Build history of the part. All positions in model axes, mm. A direction names the side the tool comes from. Round coordinates to 2 decimals unless told otherwise and drop trailing zeros. Loops run counter-clockwise (first coordinate to the right, second up) from the corner with the lowest first, then second, coordinate; pieces in that order, holes last. Notation, with made-up numbers: M 68,51.5 L 76,51.5 A23 cw 76,84.5 Z; hole C 51,-15.75 d4. An arc over 180 degrees is marked long. Use one line per item in the form item = value. Start each with the question number.
```python
from build123d import *

# Parameters (mm, degrees)
SKETCH_1_W           = 18.1
SKETCH_1_H           = 18.7
EXTRUDE_1_DEPTH      = 20
SKETCH_2_W           = 13.1
SKETCH_2_H           = 11
EXTRUDE_2_DEPTH      = 2
EXTRUDE_3_DEPTH      = 9.7
EXTRUDE_3_DEPTH_BACK = 40
FILLET_1_R           = 2.5
FILLET_2_R           = 0.5
CUT_EXTRUDE_1_DEPTH  = 49.539674531
SKETCH_5_R           = 6.105797263
CUT_EXTRUDE_2_DEPTH  = 1
SKETCH_6_R           = 6.02468661
CUT_EXTRUDE_3_DEPTH  = 1


with BuildPart() as part:
    # ｽｹｯﾁ1 → ﾎﾞｽ - 押し出し1 (new body)
    with BuildSketch(Plane.XY):
        with Locations((9.05, 9.35)):
            Rectangle(SKETCH_1_W, SKETCH_1_H)
    extrude(amount=EXTRUDE_1_DEPTH)

    # ｽｹｯﾁ2 → ﾎﾞｽ - 押し出し2 (add)
    with BuildSketch(Plane(origin=(0, 18.7, 0), x_dir=(1, 0, 0), z_dir=(0, 1, 0))):
        with Locations((9.05, -5.5)):
            Rectangle(SKETCH_2_W, SKETCH_2_H)
    extrude(amount=EXTRUDE_2_DEPTH)

    # ｽｹｯﾁ3 → ﾎﾞｽ - 押し出し3 (add, two sides: drawn at the far end of the back side and taken through both)
    with BuildSketch(Plane(origin=(0, 0, 0), x_dir=(-1, 0, 0), z_dir=(0, 0, -1)).offset(-EXTRUDE_3_DEPTH_BACK)):
        with BuildLine():
            ThreePointArc((-2.566319039, 9.311012343), (-2.144244303, 16.230296479), (-9.064933475, 15.831923002))
            ThreePointArc((-9.064933475, 15.831923002), (-15.903655717, 16.221032622), (-15.521168651, 9.381936787))
            ThreePointArc((-15.521168651, 9.381936787), (-15.948030787, 2.480748206), (-9.045010779, 2.876891972))
            ThreePointArc((-9.045010779, 2.876891972), (-2.204371262, 2.467711109), (-2.566319039, 9.311012343))
        make_face()
    extrude(amount=EXTRUDE_3_DEPTH + EXTRUDE_3_DEPTH_BACK)

    # ﾌｨﾚｯﾄ1
    fillet_1_edges = [part.edges().sort_by_distance(p)[0] for p in [
        (0, 0, 10),
        (18.1, 0, 10),
        (18.1, 18.7, 10),
        (0, 18.7, 10),
    ]]
    fillet(fillet_1_edges, radius=FILLET_1_R)

    # ﾌｨﾚｯﾄ2
    fillet_2_edges = [part.edges().sort_by_distance(p)[0] for p in [
        (0.732233047, 17.967766953, 20),
        (9.05, 18.7, 20),
        (17.367766953, 17.967766953, 20),
        (18.1, 9.35, 20),
        (17.367766953, 0.732233047, 20),
        (9.05, 0, 20),
        (0.732233047, 0.732233047, 20),
        (17.367766953, 17.967766953, 0),
        (18.1, 9.35, 0),
        (17.367766953, 0.732233047, 0),
        (9.05, 0, 0),
        (0.732233047, 0.732233047, 0),
        (0, 9.35, 0),
        (0, 9.35, 20),
        (0.732233047, 17.967766953, 0),
    ]]
    fillet(fillet_2_edges, radius=FILLET_2_R)

    # ｽｹｯﾁ4 → ｶｯﾄ - 押し出し1 (cut, through all)
    with BuildSketch(Plane(origin=(0, 0, 0), x_dir=(-1, 0, 0), z_dir=(0, 0, -1))):
        Polygon((-15.6, 18.7), (-14.085876612, 20.7), (-15.6, 20.7), align=None)
        Polygon((-2.5, 20.7), (-2.5, 18.7), (-4.014123388, 20.7), align=None)
    extrude(amount=-CUT_EXTRUDE_1_DEPTH, mode=Mode.SUBTRACT)

    # ｽｹｯﾁ5 → ｶｯﾄ - 押し出し2 (cut)
    with BuildSketch(Plane(origin=(0, 0, -9.7), x_dir=(-1, 0, 0), z_dir=(0, 0, -1))):
        with Locations((-9.054972127, 9.354407487)):
            Circle(SKETCH_5_R)
    extrude(amount=-CUT_EXTRUDE_2_DEPTH, mode=Mode.SUBTRACT)

    # ｽｹｯﾁ6 → ｶｯﾄ - 押し出し3 (cut)
    with BuildSketch(Plane.XY.offset(40)):
        with Locations((9.054972127, 9.354407487)):
            Circle(SKETCH_6_R)
    extrude(amount=-CUT_EXTRUDE_3_DEPTH, mode=Mode.SUBTRACT)


solid = part.part
```
Q1. Saw through at A-A (z = 12.5). Give the cut face in (x, y).
Q2. Saw through at D-D (y = 4). Give the cut face in (x, z), and give its area (3 significant figures).
Q3. Pull direction Y, two halves, no side cores. Call faces 4 (the face through (0, 9, 10)), 5 (the face through (10.4, 3.4, -9.2)), 6 (the face through (14.85, 19.69, 5.42)): pulls with the +Y half, pulls with the -Y half, needs draft (parallel to the pull), parting line crosses it, or undercut.
Q4. Saw through at C-C (x = 7). Give the cut face in (y, z).
Q5. Drop flat-ended pins along their axis: P1, Ø9.5, axis at x = 9.05, y = 9.35, coming from the -Z side; P2, Ø2, axis at x = 5, z = 30.5, coming from the -Y side; P3, Ø3.5, axis at x = 10.5, y = 8, coming from the +Z side. Give the stop position or say it passes through.
Q6. Tool access for faces 1 (the face through (0.713, 17.948, 10.133)), 2 (the face through (9, 17, 0)), 3 (the face through (9, 9, 39)): list every direction of +Z, -Z, +X, -X, +Y, -Y with a clear straight run to the whole face (end or side of a thin tool).
Q7. Saw through at B-B (y = 11.5). Give the cut face in (x, z).
Q8. Wall check: probe 1 along Y at (x, z) = (5.5, -4.5); probe 2 along Z at (x, y) = (7.5, 6); probe 3 along Z at (x, y) = (17.5, 12.25). Give the ranges that are in metal, low to high.
Filled in:
q1.outline = M 0,2.5 A2.5 ccw 2.5,0 L 15.6,0 A2.5 ccw 18.1,2.5 L 18.1,16.2 A2.5 ccw 15.6,18.7 L 2.5,18.7 A2.5 ccw 0,16.2 Z
q2.outline = M 0,0.5 A0.5 ccw 0.5,0 L 1.18,0 L 1.18,-9.7 L 6.12,-9.7 L 6.12,-8.7 L 11.99,-8.7 L 11.99,-9.7 L 16.95,-9.7 L 16.95,0 L 17.6,0 A0.5 ccw 18.1,0.5 L 18.1,19.5 A0.5 ccw 17.6,20 L 16.95,20 L 16.95,40 L 11.82,40 L 11.82,39 L 6.29,39 L 6.29,40 L 1.18,40 L 1.18,20 L 0.5,20 A0.5 ccw 0,19.5 Z
q2.area = 819 mm²
q3.face_4 = needs draft
q3.face_5 = undercut
q3.face_6 = pulls with the +Y half
q4.outline = M 0,0.5 A0.5 ccw 0.5,0 L 1.41,0 L 1.41,-9.7 L 3.6,-9.7 L 3.6,-8.7 L 15.1,-8.7 L 15.1,-9.7 L 17.32,-9.7 L 17.32,0 L 20.7,0 L 20.7,11 L 18.7,11 L 18.7,19.5 A0.5 ccw 18.2,20 L 17.32,20 L 17.32,40 L 15.02,40 L 15.02,39 L 3.69,39 L 3.69,40 L 1.41,40 L 1.41,20 L 0.5,20 A0.5 ccw 0,19.5 Z
q5.P1 = -8.7
q5.P2 = 1.13
q5.P3 = 39
q6.face_1 = +Z, -Z, -X, +Y
q6.face_2 = -Z
q6.face_3 = +Z
q7.outline = M 0,0.5 A0.5 ccw 0.5,0 L 1.03,0 L 1.03,-9.7 L 3.34,-9.7 L 3.34,-8.7 L 14.77,-8.7 L 14.77,-9.7 L 17.01,-9.7 L 17.01,0 L 17.6,0 A0.5 ccw 18.1,0.5 L 18.1,19.5 A0.5 ccw 17.6,20 L 17.01,20 L 17.01,40 L 14.68,40 L 14.68,39 L 3.43,39 L 3.43,40 L 1.03,40 L 1.03,20 L 0.5,20 A0.5 ccw 0,19.5 Z
q8.probe_1 = 1.13 to 17.59
q8.probe_2 = -8.7 to 39
q8.probe_3 = 0 to 20
